```python
from build123d import *

# Parameters (mm, degrees)
CROQUIS1_W              = 300
CROQUIS1_H              = 20
CROQUIS1_R              = 1.5
SALIENTE_EXTRUIR1_DEPTH = 10
CROQUIS2_W              = 240
CROQUIS2_H              = 10
SALIENTE_EXTRUIR2_DEPTH = 71
SALIENTE_EXTRUIR3_START = 10
CROQUIS3_W              = 300
CROQUIS3_H              = 20
CROQUIS3_R              = 1.5
SALIENTE_EXTRUIR3_DEPTH = 10
CROQUIS6_R              = 1.5
CORTAR_EXTRUIR1_DEPTH   = 176.72990639


with BuildPart() as part:
    # Croquis1 → Saliente-Extruir1 (new body)
    with BuildSketch(Plane.XY):
        Rectangle(CROQUIS1_W, CROQUIS1_H)
        with Locations((-139, -4)):
            Circle(CROQUIS1_R, mode=Mode.SUBTRACT)
        with Locations(Location((139, -4, 0), (0, 0, 180))):
            Circle(CROQUIS1_R, mode=Mode.SUBTRACT)
    extrude(amount=-SALIENTE_EXTRUIR1_DEPTH)

    # Croquis2 → Saliente-Extruir2 (add)
    with BuildSketch(Plane.XY):
        with Locations((0, 3.5)):
            Rectangle(CROQUIS2_W, CROQUIS2_H)
    extrude(amount=SALIENTE_EXTRUIR2_DEPTH)

    # Croquis3 → Saliente-Extruir3 (add)
    with BuildSketch(Plane.XY.offset(71).offset(SALIENTE_EXTRUIR3_START)):
        Rectangle(CROQUIS3_W, CROQUIS3_H)
        with Locations((-139, -4)):
            Circle(CROQUIS3_R, mode=Mode.SUBTRACT)
        with Locations(Location((139, -4, 0), (0, 0, 180))):
            Circle(CROQUIS3_R, mode=Mode.SUBTRACT)
    extrude(amount=-SALIENTE_EXTRUIR3_DEPTH)

    # Croquis6 → Cortar-Extruir1 (cut, through all)
    with BuildSketch(Plane(origin=(0, 0, -10), x_dir=(-1, 0, 0), z_dir=(0, 0, -1))):
        with Locations((-60.8276255, 5)):
            Circle(CROQUIS6_R)
        with Locations((60.827625106, 5.478335841)):
            Circle(CROQUIS6_R)
    extrude(amount=-CORTAR_EXTRUIR1_DEPTH, mode=Mode.SUBTRACT)


solid = part.part
```
CAD build for the part. Positions are in the model's coordinates, mm. A direction names the side the tool comes from. Coordinates: 2 decimals unless noted, no trailing zeros. Write each loop counter-clockwise with the first axis right and the second up, starting at its lowest first coordinate (ties: lowest second). Pieces come first, ordered by that corner, then holes. Notation, with made-up numbers: (-35, 48) -> (-20, 48) arc R9 ccw to (-20, 65) -> close; hole circle Ø6 at (86.25, 82). An arc over 180 degrees is marked (long way). Use CSV: the item, a comma, the result in double quotes. Start each with the question number.
Item 1: Band-saw the part on A-A, the plane x = 66. Write the cut outline in (y, z), plus the area to 3 significant figures.
Item 2: Wall check: probe 1 along X at (y, z) = (5.25, 59); probe 2 along Z at (x, y) = (129, 7.75); probe 3 along Y at (x, z) = (-139, 74.75). Give the ranges that are in metal, low to high.
Item 3: Tool access for faces 1 (the flat face through (-120, 3, 35)), 2 (the flat face through (120, 3, 35)), 3 (the flat face through (-2, 8.5, 35)), 4 (the flat face through (-2, -1.5, 35)), 5 (the flat face through (-150, 0, -5)): list every direction of +Z, -Z, +X, -X, +Y, -Y with a clear straight run to the whole face (end or side of a thin tool).
Item 4: Drop flat-ended pins along their axis: P1, Ø1, axis at x = 90, z = 54, coming from the +Y side; P2, Ø11, axis at y = 3.5, z = 51, coming from the +X side; P3, Ø11, axis at y = 3, z = 30.5, coming from the -X side. Give the stop position or say it passes through.
Item 5: Band-saw the part on B-B, the plane z = 22. Write the cut outline in (x, y), plus the area to 3 significant figures.
Response values:
1,outline,"(-10, -10) -> (10, -10) -> (10, 0) -> (8.5, 0) -> (8.5, 71) -> (10, 71) -> (10, 81) -> (-10, 81) -> (-10, 71) -> (-1.5, 71) -> (-1.5, 0) -> (-10, 0) -> close"
1,area,"1,110 mm2"
2,probe 1,"x = -120 to -62.31, -59.35 to 59.35, 62.31 to 120"
2,probe 2,"z = -10 to 0, 71 to 81"
2,probe 3,"y = -10 to -5.5, -2.5 to 10"
3,face 1,"-X, +Y, -Y"
3,face 2,"+X, +Y, -Y"
3,face 3,"+X, -X, +Y"
3,face 4,"+X, -X, -Y"
3,face 5,"+Z, -Z, -X, +Y, -Y"
4,P1,"stops at y = 8.5"
4,P2,"stops at x = 120"
4,P3,"stops at x = -120"
5,outline,"(-120, -1.5) -> (120, -1.5) -> (120, 8.5) -> (-120, 8.5) -> close; hole circle Ø3 at (-60.83, 5.48); hole circle Ø3 at (60.83, 5)"
5,area,"2,390 mm2"
